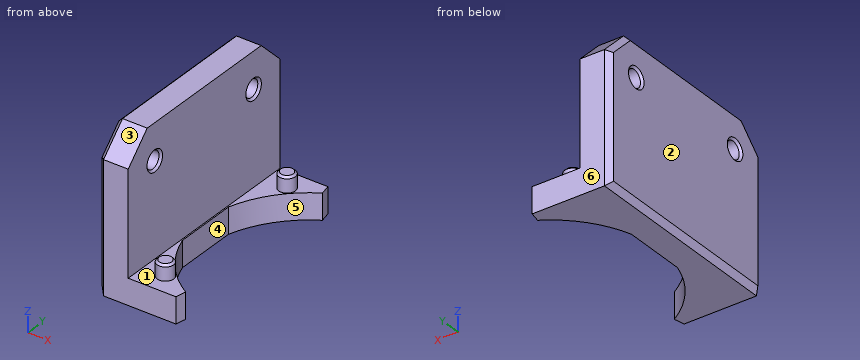
from build123d import *

# Parameters (mm, degrees)
SKETCH105_W              = 21
SKETCH105_H              = 40
PAD032_DEPTH             = 30
POCKET067_DEPTH          = 5
SKETCH107_W              = 20.25
SKETCH107_H              = 40
POCKET068_DEPTH          = 25
SKETCH108_R              = 1.6
PAD033_DEPTH             = 3
SKETCH109_R              = 1.65
POCKET069_DEPTH          = 19.933875
CHAMFER009002001006_SIZE = 5
CHAMFER009002001007_SIZE = 5
CHAMFER009002001008_SIZE = 1
CHAMFER009002001009_SIZE = 0.4


with BuildPart() as part:
    # Sketch105 → Pad032 (new body)
    with BuildSketch(Plane.XY):
        with Locations((-15.5, 0)):
            Rectangle(SKETCH105_W, SKETCH105_H)
    extrude(amount=PAD032_DEPTH)

    # Sketch106 (on Face5 of Pad032) → Pocket067 (cut)
    with BuildSketch(Plane(origin=(0, 0, 0), x_dir=(1, 0, 0), z_dir=(0, 0, -1))):
        with BuildLine():
            ThreePointArc((-20, -6.067125), (20.9, 0), (-20, 6.067125))
            Line((-20, 6.067125), (-20, -6.067125))
        make_face()
    extrude(amount=-POCKET067_DEPTH, mode=Mode.SUBTRACT)

    # Sketch107 (on Face6 of Pocket067) → Pocket068 (cut)
    with BuildSketch(Plane.XY.offset(30)):
        with Locations((-10.125, 0)):
            Rectangle(SKETCH107_W, SKETCH107_H)
    extrude(amount=-POCKET068_DEPTH, mode=Mode.SUBTRACT)

    # Sketch108 (on Face4 of Pocket068) → Pad033 (join)
    with BuildSketch(Plane.XY.offset(5)):
        with Locations((-16, 16)):
            Circle(SKETCH108_R)
        with Locations((-16, -16)):
            Circle(SKETCH108_R)
    extrude(amount=PAD033_DEPTH)

    # Sketch109 (on Face7 of Pad033) → Pocket069 (cut, through all)
    with BuildSketch(Plane(origin=(-26, 0, 0), x_dir=(0, -1, 0), z_dir=(-1, 0, 0))):
        with Locations((-13, 23)):
            Circle(SKETCH109_R)
        with Locations((13, 23)):
            Circle(SKETCH109_R)
    extrude(amount=-POCKET069_DEPTH, mode=Mode.SUBTRACT)

    # Chamfer009002001006
    chamfer009002001006_edges = [part.edges().sort_by_distance(p)[0] for p in [
        (-23.125, 20, 30),
        (-23.125, -20, 30),
    ]]
    chamfer(chamfer009002001006_edges, length=CHAMFER009002001006_SIZE)

    # Chamfer009002001007
    chamfer009002001007_edges = [part.edges().sort_by_distance(p)[0] for p in [
        (-6.067125, -20, 2.5),
        (-6.067125, 20, 2.5),
    ]]
    chamfer(chamfer009002001007_edges, length=CHAMFER009002001007_SIZE)

    # Chamfer009002001008
    chamfer009002001008_edges = [part.edges().sort_by_distance(p)[0] for p in [
        (-26, 0, 0),
        (-26, 20, 12.5),
        (-26, 17.5, 27.5),
        (-26, 0, 30),
        (-26, -17.5, 27.5),
        (-26, -20, 12.5),
    ]]
    chamfer(chamfer009002001008_edges, length=CHAMFER009002001008_SIZE)

    # Chamfer009002001009
    chamfer009002001009_edges = [part.edges().sort_by_distance(p)[0] for p in [
        (-26, 14.65, 23),
        (-26, -11.35, 23),
        (-17.6, -16, 8),
        (-17.6, 16, 8),
        (-20.25, 14.65, 23),
        (-20.25, -11.35, 23),
    ]]
    chamfer(chamfer009002001009_edges, length=CHAMFER009002001009_SIZE)


with BuildPart() as part_1:
    # Body012 placement: moved
    add(part.part.moved(Location((0, 0, -10))))


solid = part_1.part
Build history of the part. All positions in model axes, mm. Face numbers are marked on the shaded views. A direction names the side the tool comes from. Give positions to 0.01 mm unless a question says otherwise; leave off trailing zeros. Loops run counter-clockwise (first coordinate to the right, second up) from the corner with the lowest first, then second, coordinate; pieces in that order, holes last. Notation, with made-up numbers: (15, 33.25) -> (50, 33.25) arc R21 cw to (50, 57.25) -> close; hole circle Ø2 at (-31.5, 71.25). An arc over 180 degrees is marked (long way). Answer in a Markdown table with one row per item.
Item 1: Slice it at C-C on y = -0.5. Write the cut outline in (x, z), plus the area to 3 significant figures.
Findings below:
| item | result |
|---|---|
| outline | (-26, -9) -> (-25, -10) -> (-20, -10) -> (-20, -5) -> (-20.25, -5) -> (-20.25, 20) -> (-25, 20) -> (-26, 19) -> close |
| area | 173 mm² |
Item 2: Tool access for the marked faces 1 and 2: list every direction of +Z, -Z, +X, -X, +Y, -Y with a clear straight run to the whole face (end or side of a thin tool).
Findings below:
| item | result |
|---|---|
| face 1 | +Z |
| face 2 | +Z, -Z, -X, +Y, -Y |
Item 3: Slice it at A-A on x = -22.5. Write the cut outline in (y, z).
Findings below:
| item | result |
|---|---|
| outline | (-20, -10) -> (20, -10) -> (20, 15) -> (15, 20) -> (-15, 20) -> (-20, 15) -> close; hole circle Ø3.3 at (-13, 13); hole circle Ø3.3 at (13, 13) |
Item 4: Slice it at D-D on x = -16. Write the cut outline in (y, z).
Findings below:
| item | result |
|---|---|
| outline | (-20, -10) -> (-13.45, -10) -> (-13.45, -5) -> (-14.4, -5) -> (-14.4, -2.4) -> (-14.8, -2) -> (-17.2, -2) -> (-17.6, -2.4) -> (-17.6, -5) -> (-20, -5) -> close; (13.45, -10) -> (20, -10) -> (20, -5) -> (17.6, -5) -> (17.6, -2.4) -> (17.2, -2) -> (14.8, -2) -> (14.4, -2.4) -> (14.4, -5) -> (13.45, -5) -> close |
Item 5: Probe line 1 along Z through (x, y) = (-22.3, -13); line 2 along X through (y, z) = (-2, -4.5); line 3 along Z through (x, y) = (-18.5, 17). List the from-to ranges inside material, lowest first. Write a range as [from, to].
Findings below:
| item | result |
|---|---|
| line 1 | z = [-10, 11.35], [14.65, 20] |
| line 2 | x = [-26, -20.25] |
| line 3 | z = [-10, -5] |
Item 6: Flat gauge pins, fed straight in: P1, Ø5.5, axis at y = 13, z = 13, coming from the +X side; P2, Ø3, axis at x = -16, y = 15, coming from the +Z side; P3, Ø2.5, axis at y = 0.5, z = -7, coming from the +X side. Where does each tip first touch, or does it go through?
Findings below:
| item | result |
|---|---|
| P1 | stops at x = -20.25 |
| P2 | stops at z = -2 |
| P3 | stops at x = -20 |
Item 7: Mould opens along Y. For the marked faces 3, 4, 5 and 6 say: pulls with the +Y half, pulls with the -Y half, needs draft (parallel to the pull), parting line crosses it, or undercut.
Findings below:
| item | result |
|---|---|
| face 3 | pulls with the -Y half |
| face 4 | undercut |
| face 5 | undercut |
| face 6 | pulls with the +Y half |
Item 8: Slice it at B-B on z = -4.25. Write the cut outline in (x, y), plus the area to 3 significant figures.
Findings below:
| item | result |
|---|---|
| outline | (-26, -19) -> (-25, -20) -> (-20.25, -20) -> (-20.25, 20) -> (-25, 20) -> (-26, 19) -> close; circle Ø3.2 at (-16, -16); circle Ø3.2 at (-16, 16) |
| area | 245 mm² |
